```python
from build123d import *

# Parameters (mm, degrees)
F1_DEPTH = 6.35


# Not quite as in the source:
# - ends of sketch curves that miss each other by under 0.0002 mm in the source are joined


with BuildPart() as f1:
    # F0 (on Top) → F1 (new body)
    with BuildSketch(Plane.XY):
        with BuildLine():
            Line((-111.08563, 71.3839822), (-70.59041, -68.9586378))
            ThreePointArc((-70.59041, -68.9586378), (-0.3347578994, -121.8821648179), (70.0620962947, -69.1465996345))
            Line((70.0620962947, -69.1465996345), (111.08563, 71.6151222))
            ThreePointArc((111.08563, 71.6151222), (98.7152655637, 104.8392134799), (67.6282616967, 121.882228124))
            Line((67.6282616967, 121.882228124), (67.628262, 75.5002554))
            ThreePointArc((67.628262, 75.5002554), (57.7977885358, 70.4247346397), (47.5906584666, 66.156994374))
            ThreePointArc((47.5906584666, 66.156994374), (-0.23749, 33.3973424), (-48.0656463013, 66.1569896482))
            ThreePointArc((-48.0656463013, 66.1569896482), (-58.2727685358, 70.4247346397), (-68.1032374015, 75.5002634895))
            Line((-68.1032374015, 75.5002634895), (-68.103242, 121.5776334))
            ThreePointArc((-68.103242, 121.5776334), (-98.8713942195, 104.4249578962), (-111.08563, 71.3839822))
        make_face()
        with BuildLine():
            ThreePointArc((-6.58749, -108.1531492), (-0.23749, -101.8031492), (6.11251, -108.1531492))
            ThreePointArc((6.11251, -108.1531492), (-0.23749, -114.5031492), (-6.58749, -108.1531492))
        make_face(mode=Mode.SUBTRACT)
        with BuildLine():
            ThreePointArc((-66.0816814, -48.6589578), (-59.7316814, -42.3089578), (-53.3816814, -48.6589578))
            ThreePointArc((-53.3816814, -48.6589578), (-59.7316814, -55.0089578), (-66.0816814, -48.6589578))
        make_face(mode=Mode.SUBTRACT)
        with BuildLine():
            ThreePointArc((-48.65624, -48.6589578), (-0.23749, -0.2402078), (48.18126, -48.6589578))
            ThreePointArc((48.18126, -48.6589578), (-0.23749, -97.0777078), (-48.65624, -48.6589578))
        make_face(mode=Mode.SUBTRACT)
        with BuildLine():
            ThreePointArc((52.9067014, -48.6589578), (59.2567014, -42.3089578), (65.6067014, -48.6589578))
            ThreePointArc((65.6067014, -48.6589578), (59.2567014, -55.0089578), (52.9067014, -48.6589578))
        make_face(mode=Mode.SUBTRACT)
        with BuildLine():
            ThreePointArc((-6.58749, 10.8352336), (-0.23749, 17.1852336), (6.11251, 10.8352336))
            ThreePointArc((6.11251, 10.8352336), (-0.23749, 4.4852336), (-6.58749, 10.8352336))
        make_face(mode=Mode.SUBTRACT)
        with BuildLine():
            ThreePointArc((-94.69374, 90.8966432), (-89.93124, 95.6591432), (-85.16874, 90.8966432))
            ThreePointArc((-85.16874, 90.8966432), (-89.93124, 86.1341432), (-94.69374, 90.8966432))
        make_face(mode=Mode.SUBTRACT)
        with BuildLine():
            ThreePointArc((84.69376, 90.8966432), (89.45626, 95.6591432), (94.21876, 90.8966432))
            ThreePointArc((94.21876, 90.8966432), (89.45626, 86.1341432), (84.69376, 90.8966432))
        make_face(mode=Mode.SUBTRACT)
    extrude(amount=F1_DEPTH)


solid = f1.part
```
The model under review builds one solid part; all positions refer to its coordinate system, in mm. A direction names the side the tool comes from. Round coordinates to 2 decimals unless told otherwise and drop trailing zeros. Loops run counter-clockwise (first coordinate to the right, second up) from the corner with the lowest first, then second, coordinate; pieces in that order, holes last. Notation, with made-up numbers: M 18,57 L 67,57 A17 cw 67,70 Z; hole C 67.5,-2 d6. An arc over 180 degrees is marked long. Put each result on its own line as item: value.
Q1. Consider section C-C, the plane y = -45.5. Give the boundary of the cut face in (x, z), then the cut area to 3 significant figures.
Result set:
outline: M -77.36,0 L -65.24,0 L -65.24,6.35 L -77.36,6.35 Z; M -54.22,0 L -48.55,0 L -48.55,6.35 L -54.22,6.35 Z; M 48.08,0 L 53.75,0 L 53.75,6.35 L 48.08,6.35 Z; M 64.77,0 L 76.95,0 L 76.95,6.35 L 64.77,6.35 Z
area: 226 mm²
Q2. Machinability: for faces 5 (the cylindrical face through (-90.551, 86.175, 3.131)), 6 (the cylindrical face through (57.94, 70.49, 3.13)), which of the approach directions +Z, -Z, +X, -X, +Y, -Y give a long, thin tool a straight path to every point of the face, cutting with its end or side? Answer none if there is none.
Result set:
face 5: +Z, -Z
face 6: +Z, -Z, +Y
Q3. For pin 1 (1.5 mm diameter, centred on x = 83.5, z = 1, fed in from +Y); pin 2 (3 mm diameter, centred on y = 94, z = 3, fed in from +X); pin 3 (1.5 mm diameter, centred on x = 66, z = 2.5, fed in from +Y), all flat-tipped, find the tip position at first contact; note any pin that passes through.
Result set:
pin 1: stops at y = 117.18
pin 2: stops at x = 106.59
pin 3: stops at y = 75.01
Q4. To check wall thickness, follow L1, parallel to Y at x = -3, z = 3.5; L2, parallel to X at y = 95, z = 1.5; L3, parallel to X at y = 12, z = 4.5. State the ranges of each line that lie inside material, in increasing order.
Result set:
L1: y = -121.83 to -113.87, -102.44 to -97, -0.32 to 5.12, 16.55 to 33.47
L2: x = -105.26 to -92.35, -87.51 to -68.1, 67.63 to 87.04, 91.87 to 105.38
L3: x = -93.95 to -6.48, 6 to 93.71
Q5. Consider section B-B, the plane x = -26.5. Give the boundary of the cut face in (y, z), then the cut area to 3 significant figures.
Result set:
outline: M -117.01,0 L -89.34,0 L -89.34,6.35 L -117.01,6.35 Z; M -7.98,0 L 40.63,0 L 40.63,6.35 L -7.98,6.35 Z
area: 484 mm²
Q6. Mouldability with a two-part tool opening along X and no side actions: class faces 1 (the cylindrical face through (-1.66, -121.87, 3.13)), 2 (the flat face through (-91.121, 2.195, 3.131)), 3 (the flat face through (-2, 2, 6.35)), 4 (the cylindrical face through (-1.614, 17.034, 3.131)) as released by +X, released by -X, zero draft, split by the parting line, or undercut.
Result set:
face 1: split by the parting line
face 2: released by -X
face 3: zero draft
face 4: undercut
Q7. Consider section A-A, the plane y = -80. Give the boundary of the cut face in (x, z), then the cut area to 3 significant figures.
Result set:
outline: M -66.41,0 L -37.14,0 L -37.14,6.35 L -66.41,6.35 Z; M 36.67,0 L 65.94,0 L 65.94,6.35 L 36.67,6.35 Z
area: 372 mm²
Q8. Consider section D-D, the plane z = 3.5. Count the separate pieces of the cut face and the enclosed holes in it, then the cut area to 3 significant figures.
Result set:
separate pieces: 1
enclosed holes: 7
area: 23,400 mm²
